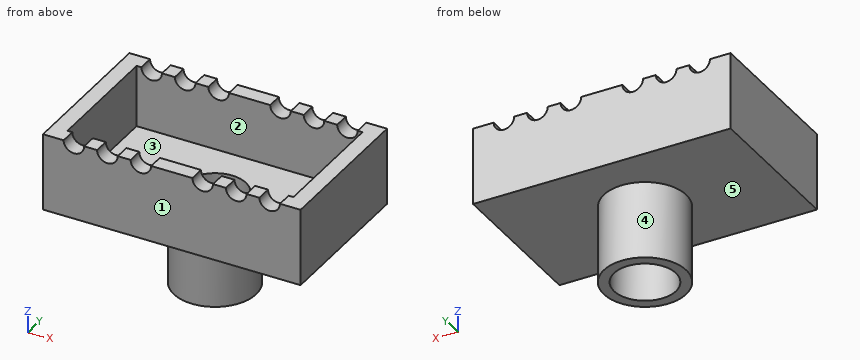
```python
from build123d import *

# Parameters (mm, degrees)
F0_W          = 50
F0_H          = 30
F0_W_2        = 43.8518549643
F0_H_2        = 24
F1_DEPTH      = 15
F0_R          = 8
F2_DEPTH      = 3
F0_R_2        = 6
F3_DEPTH      = 15
F3_DEPTH_BACK = 3
F5_DEPTH      = 46.6


with BuildPart() as f1:
    # F0 (on Top) → F1 (new body)
    with BuildSketch(Plane.XY):
        Rectangle(F0_W, F0_H)
        Rectangle(F0_W_2, F0_H_2, mode=Mode.SUBTRACT)
    extrude(amount=F1_DEPTH)

    # F0 (on Top) → F2 (join)
    with BuildSketch(Plane.XY):
        Rectangle(F0_W_2, F0_H_2)
        Circle(F0_R, mode=Mode.SUBTRACT)
    extrude(amount=F2_DEPTH)

    # F0 (on Top) → F3 (join, two sides)
    with BuildSketch(Plane.XY) as f3_sk:
        Circle(F0_R)
        Circle(F0_R_2, mode=Mode.SUBTRACT)
    extrude(amount=-F3_DEPTH)
    extrude(f3_sk.sketch, amount=F3_DEPTH_BACK)

    # F4 (on face) → F5 (cut)
    with BuildSketch(Plane.XZ.offset(15)):
        with BuildLine():
            ThreePointArc((-17, 15), (-19, 17), (-21, 15))
            Line((-21, 15), (-17, 15))
        make_face()
        with BuildLine():
            ThreePointArc((21, 15), (19, 17), (17, 15))
            Line((17, 15), (21, 15))
        make_face()
        with BuildLine():
            Line((21, 15), (17, 15))
            ThreePointArc((17, 15), (19, 13), (21, 15))
        make_face()
        with BuildLine():
            ThreePointArc((14.5, 15), (12.5, 17), (10.5, 15))
            Line((10.5, 15), (14.5, 15))
        make_face()
        with BuildLine():
            Line((14.5, 15), (10.5, 15))
            ThreePointArc((10.5, 15), (12.5, 13), (14.5, 15))
        make_face()
        with BuildLine():
            ThreePointArc((8, 15), (6, 17), (4, 15))
            Line((4, 15), (8, 15))
        make_face()
        with BuildLine():
            Line((8, 15), (4, 15))
            ThreePointArc((4, 15), (6, 13), (8, 15))
        make_face()
        with BuildLine():
            ThreePointArc((-4, 15), (-6, 17), (-8, 15))
            Line((-8, 15), (-4, 15))
        make_face()
        with BuildLine():
            Line((-4, 15), (-8, 15))
            ThreePointArc((-8, 15), (-6, 13), (-4, 15))
        make_face()
        with BuildLine():
            ThreePointArc((-10.5, 15), (-12.5, 17), (-14.5, 15))
            Line((-14.5, 15), (-10.5, 15))
        make_face()
        with BuildLine():
            Line((-10.5, 15), (-14.5, 15))
            ThreePointArc((-14.5, 15), (-12.5, 13), (-10.5, 15))
        make_face()
        with BuildLine():
            Line((-17, 15), (-21, 15))
            ThreePointArc((-21, 15), (-19, 13), (-17, 15))
        make_face()
    extrude(amount=-F5_DEPTH, mode=Mode.SUBTRACT)


solid = f1.part
```
Read the model definition and answer for the solid it produces. Units are mm, in the model's axes. Face numbers are marked on the shaded views. A direction names the side the tool comes from. Give positions to 0.01 mm unless a question says otherwise; leave off trailing zeros. Write each loop counter-clockwise with the first axis right and the second up, starting at its lowest first coordinate (ties: lowest second). Pieces come first, ordered by that corner, then holes. Notation, with made-up numbers: (1, 28.25) - (11, 28.25) arc R22 ccw to (11, 45.25) - close; hole circle Ø1 at (-11, 52.5). An arc over 180 degrees is marked (long way). Write item = value, one per line. Start each with the question number.
Item 1: Find section C-C (y = -9.75). Give the vertices of the cut face in (x, z).
Item 2: Each of these flat-tipped pins is pushed along its axis until it touches: P1, Ø2, axis at x = -15, y = 5, coming from the -Z side; P2, Ø14, axis at x = 0, y = 0, coming from the +Z side; P3, Ø3, axis at y = 1, z = -2, coming from the -X side. Where does it stop, or does it pass through?
Item 3: Find section B-B (z = 4.5). Give the vertices of the cut face in (x, y), then the cut area to 3 significant figures.
Item 4: Find section D-D (x = -19). Give the vertices of the cut face in (y, z), then the cut area to 3 significant figures.
Item 5: Find the intervals of material crossed by probe 1 along Y at (x, z) = (0, -2); probe 2 along Y at (x, z) = (1.5, 10); probe 3 along X at (y, z) = (4.5, 8), in increasing order. Write a range as [from, to].
Item 6: A tool of negligible diameter and unlimited length cuts with its end or side. For the marked faces 1 and 2, from which of +Z, -Z, +X, -X, +Y, -Y can it reach the whole face along a straight path? Write none if from no direction.
Item 7: Find section A-A (x = 0). Give the vertices of the cut face in (y, z).
Item 8: The mould has two halves that part along Y. Classify the marked faces 3, 4 and 5: +Y half, -Y half, draft (parallel to the pull), parting line (faces both ways), or undercut.
Response:
q1.outline = (-25, 0) - (25, 0) - (25, 15) - (21.93, 15) - (21.93, 3) - (-21.93, 3) - (-21.93, 15) - (-25, 15) - close
q2.P1 = 0
q2.P2 = 3
q2.P3 = -8
q3.outline = (-25, -15) - (25, -15) - (25, 15) - (-25, 15) - close; hole (-21.93, -12) - (21.93, -12) - (21.93, 12) - (-21.93, 12) - close
q3.area = 448 mm²
q4.outline = (-15, 0) - (15, 0) - (15, 13) - (12, 13) - (12, 3) - (-12, 3) - (-12, 13) - (-15, 13) - close
q4.area = 150 mm²
q5.probe_1 = [-8, -6], [6, 8]
q5.probe_2 = [-15, -12], [12, 15]
q5.probe_3 = [-25, -21.93], [21.93, 25]
q6.face_1 = +Z, -Z, +X, -X, -Y
q6.face_2 = +Z
q7.outline = (-15, 0) - (-8, 0) - (-8, -15) - (-6, -15) - (-6, 3) - (-12, 3) - (-12, 15) - (-15, 15) - close; (6, -15) - (8, -15) - (8, 0) - (15, 0) - (15, 15) - (12, 15) - (12, 3) - (6, 3) - close
q8.face_3 = undercut
q8.face_4 = parting line
q8.face_5 = draft
